Design review of the part built by this model. Coordinates are the model's own, in mm. A direction names the side the tool comes from. Coordinates: 2 decimals unless noted, no trailing zeros. Loops run counter-clockwise (first coordinate to the right, second up) from the corner with the lowest first, then second, coordinate; pieces in that order, holes last. Notation, with made-up numbers: M 60,-32.5 L 107,-32.5 A8 cw 107,-27.5 Z; hole C 57,45 d6. An arc over 180 degrees is marked long. Write item = value, one per line. Start each with the question number.
from build123d import *

# Parameters (mm, degrees)
F2_DEPTH = 10
F3_R     = 2.15
F4_DEPTH = 25


with BuildPart() as f2:
    # F1 (on Front) → F2 (new body)
    with BuildSketch(Plane.XZ):
        with BuildLine():
            Line((-25.5, -3.4), (-25.5, -8.4))
            Line((-25.5, -8.4), (-8.5, -8.4))
            Line((-8.5, -8.4), (-8.5, 0))
            ThreePointArc((-8.5, 0), (-6.0104076434, 6.0104076368), (-9.4e-09, 8.5))
            Line((-9.4e-09, 8.5), (-10.4880884817, 8.5))
            ThreePointArc((-10.4880884817, 8.5), (-12.7247631511, 4.5089247885), (-13.5, 0))
            Line((-13.5, 0), (-13.5, -3.4))
            Line((-13.5, -3.4), (-25.5, -3.4))
        make_face()
        with BuildLine():
            Line((10.4880884817, 8.5), (-9.4e-09, 8.5))
            ThreePointArc((-9.4e-09, 8.5), (6.0104076368, 6.0104076434), (8.5, 0))
            Line((8.5, 0), (8.5, -8.4))
            Line((8.5, -8.4), (25.5, -8.4))
            Line((25.5, -8.4), (25.5, -3.4))
            Line((25.5, -3.4), (13.5, -3.4))
            Line((13.5, -3.4), (13.5, 0))
            ThreePointArc((13.5, 0), (12.7247631511, 4.5089247885), (10.4880884817, 8.5))
        make_face()
        with BuildLine():
            Line((-10.4880884817, 8.5), (-9.4e-09, 8.5))
            Line((-9.4e-09, 8.5), (10.4880884817, 8.5))
            ThreePointArc((10.4880884817, 8.5), (0, 13.5), (-10.4880884817, 8.5))
        make_face()
        with BuildLine():
            Line((-25.5, 8.5), (-10.4880884817, 8.5))
            ThreePointArc((-10.4880884817, 8.5), (0, 13.5), (10.4880884817, 8.5))
            Line((10.4880884817, 8.5), (25.5, 8.5))
            Line((25.5, 8.5), (25.5, 15.6))
            Line((25.5, 15.6), (-25.5, 15.6))
            Line((-25.5, 15.6), (-25.5, 8.5))
        make_face()
    extrude(amount=F2_DEPTH)

    # F3 (on Top) → F4 (cut, symmetric)
    with BuildSketch(Plane.XY):
        with Locations((-21.15, -5)):
            Circle(F3_R)
        with Locations((21.15, -5)):
            Circle(F3_R)
    extrude(amount=F4_DEPTH, both=True, mode=Mode.SUBTRACT)


solid = f2.part
Q1. Add section B-B on x = -21.15. State the section outline as (y, z) points, plus the area to 3 significant figures.
Q2. Clearance check with flat-ended pins moving along their axes: P1, Ø1.7, axis at y = -3, z = -2, coming from the +X side; P2, Ø2.5, axis at y = -3, z = -1, coming from the -X side. State where each tip first meets the part, or that it passes through.
Q3. Add section C-C on y = -8.75. State the section outline as (x, z) points.
Q4. Mouldability with a two-part tool opening along Z and no side actions: class faces 6 (the face through (17, -5, -8.4)), 7 (the face through (-18, -5, 8.5)), 8 (the face through (19, -5, 12)), 9 (the face through (0, -5, 15.6)) as released by +Z, released by -Z, zero draft, split by the parting line, or undercut.
Q5. Add section A-A on z = -5.25. State the section outline as (x, y) points.
Q6. To check wall thickness, follow line 1 (X direction, y = -9.5, z = -4.5); line 2 (X direction, y = -3.75, z = -0.5); line 3 (Z direction, x = 15.5, y = -0.5). State the ranges of each line that lie inside material, in increasing order. Write a range as from..to.
Q7. For faces 1 (the face through (-19.1, -4.35, -5.86)), 2 (the face through (18, -5, 8.5)), 3 (the face through (8.5, -5, -4)), 4 (the face through (-13.5, -5, -2)), 5 (the face through (25.5, -5, -6)), list the 3-axis set-ups (+Z, -Z, +X, -X, +Y, -Y) from which the entire face can be reached by the end or side of a thin tool; tool diameter is ignored.
Q8. Add section D-D on z = 7.75. State the section outline as (x, y) points, plus the area to 3 significant figures.
Values follow:
q1.outline = M -10,-8.4 L -7.15,-8.4 L -7.15,-3.4 L -10,-3.4 Z; M -10,8.5 L -7.15,8.5 L -7.15,15.6 L -10,15.6 Z; M -2.85,-8.4 L 0,-8.4 L 0,-3.4 L -2.85,-3.4 Z; M -2.85,8.5 L 0,8.5 L 0,15.6 L -2.85,15.6 Z
q1.area = 69.0 mm2
q2.P1 = 13.5
q2.P2 = -13.5
q3.outline = M -25.5,-8.4 L -8.5,-8.4 L -8.5,0 A8.5 cw 8.5,0 L 8.5,-8.4 L 25.5,-8.4 L 25.5,-3.4 L 13.5,-3.4 L 13.5,0 A13.5 ccw 10.49,8.5 L 25.5,8.5 L 25.5,15.6 L -25.5,15.6 L -25.5,8.5 L -10.49,8.5 A13.5 ccw -13.5,0 L -13.5,-3.4 L -25.5,-3.4 Z
q4.face_6 = released by -Z
q4.face_7 = undercut
q4.face_8 = zero draft
q4.face_9 = released by +Z
q5.outline = M -25.5,-10 L -8.5,-10 L -8.5,0 L -25.5,0 Z; M 8.5,-10 L 25.5,-10 L 25.5,0 L 8.5,0 Z; hole C -21.15,-5 d4.3; hole C 21.15,-5 d4.3
q6.line_1 = -25.5..-8.5, 8.5..25.5
q6.line_2 = -13.5..-8.5, 8.5..13.5
q6.line_3 = -8.4..-3.4, 8.5..15.6
q7.face_1 = +Z, -Z
q7.face_2 = +X, +Y, -Y
q7.face_3 = -Z, +Y, -Y
q7.face_4 = -X, +Y, -Y
q7.face_5 = +Z, -Z, +X, +Y, -Y
q8.outline = M -11.05,-10 L -3.49,-10 L -3.49,0 L -11.05,0 Z; M 3.49,-10 L 11.05,-10 L 11.05,0 L 3.49,0 Z
q8.area = 151 mm2
